Could you check a few things on this model? Use its own coordinates, in mm. Face numbers are marked on the shaded views. A direction names the side the tool comes from. Give positions to 0.01 mm unless a question says otherwise; leave off trailing zeros. Write each loop counter-clockwise with the first axis right and the second up, starting at its lowest first coordinate (ties: lowest second). Pieces come first, ordered by that corner, then holes. Notation, with made-up numbers: (82, 20.5) - (96, 20.5) arc R26 cw to (96, 47.5) - close; hole circle Ø5 at (33, -4.5). An arc over 180 degrees is marked (long way). Answer as CSV lines item,"result". Start each with the question number.
Q1. Will these pins go through, and if not, where does the flat tip stop? pin 1 Ø1.5 at (x, z) = (2.5, 4) entering from +Y; pin 2 Ø2 at (x, z) = (9.5, 3.5) entering from +Y; pin 3 Ø2 at (x, z) = (11.5, 14) entering from -Y.
Q2. Imagine slicing it at C-C on z = 22.5. List the corners of the cut face in (x, y) for me, and give its area (3 significant figures).
Q3. On a 3-axis mill with a long thin cutter (end or side, diameter ignored), from which of +Z, -Z, +X, -X, +Y, -Y can I reach the whole of each face in a straight line? I mean the marked faces 4, 5 and 6. Say none if no direction works.
Q4. We'd pull the mould along Y, two halves only. Please class the marked faces 1, 2 and 3: pulls with the +Y half, pulls with the -Y half, needs draft (parallel to the pull), parting line crosses it, or undercut.
Q5. Imagine slicing it at A-A on z = 10.5. List the corners of the cut face in (x, y) for me.
Q6. Imagine slicing it at D-D on x = 8.5. List the corners of the cut face in (y, z) for me, and give its area (3 significant figures).
Q7. If I drill on line 1 along Y through (x, z) = (0, 4); line 2 along X through (y, z) = (0, 5); line 3 along Y through (x, z) = (-5, 19.25), over which ranges is the centre line in solid material (lowest first)?
```python
from build123d import *

# Parameters (mm, degrees)
F0_R     = 15
F1_DEPTH = 9
F2_R     = 0.5
F3_DEPTH = 10
F6_DEPTH = 5


# Not quite as in the source:
# - a fillet or chamfer that OpenCascade refuses, or shapes differently, is made with other operations: its cross-section is extruded or revolved along the edge and cut away or added


with BuildPart() as f1:
    # F0 (on Top) → F1 (new body)
    with BuildSketch(Plane.XY):
        Circle(F0_R)
        with BuildLine():
            Line((-2.2, -2.3237900077), (-2.2, 2.3237900077))
            ThreePointArc((-2.2, 2.3237900077), (3.2, 0), (-2.2, -2.3237900077))
        make_face(mode=Mode.SUBTRACT)
    extrude(amount=F1_DEPTH)

    # F2 (on face) → F3 (join)
    with BuildSketch(Plane.XY.offset(9)):
        with BuildLine():
            Line((-7, 6), (-15, 0))
            Line((-15, 0), (-7, -6))
            Line((-7, -6), (13.7477270849, -6))
            ThreePointArc((13.7477270849, -6), (14.683594694, -3.0646446553), (15, 0))
            ThreePointArc((15, 0), (14.683594694, 3.0646446553), (13.7477270849, 6))
            Line((13.7477270849, 6), (-7, 6))
        make_face()
        Circle(F2_R, mode=Mode.SUBTRACT)
    extrude(amount=F3_DEPTH)

    # F4: chamfer of 10 x 2.6794919243 on 1 edges, made by hand


with BuildPart() as f4_tool2:
    # F4_s3 → F4_t4 (revolve)
    with BuildSketch(Plane.XZ):
        Polygon((3.1794919243, 9), (0.5, 19), (0.5, 9), align=None)
    revolve(axis=Axis((0, 0, 9), (0, 0, 1)))

    split(bisect_by=Plane.YZ.offset(-2.2), keep=Keep.TOP)


with BuildPart() as f1_1:
    add(f1.part)

    # F4_t1: cut F4_tool2
    add(f4_tool2.part, mode=Mode.SUBTRACT)

    # F5 (on face) → F6 (join)
    with BuildSketch(Plane.XY.offset(19)):
        with BuildLine():
            Line((-7, 6), (-15, 0))
            Line((-15, 0), (-7, -6))
            Line((-7, -6), (13.7477270849, -6))
            ThreePointArc((13.7477270849, -6), (15, 0), (13.7477270849, 6))
            Line((13.7477270849, 6), (-7, 6))
        make_face()
    extrude(amount=F6_DEPTH)


solid = f1_1.part
```
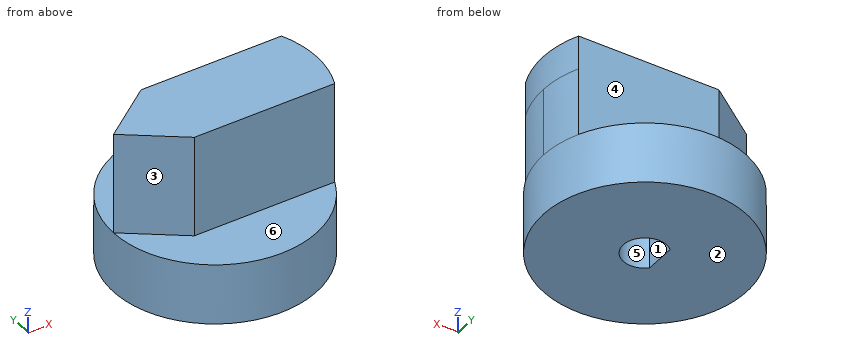
Conclusion:
1,pin 1,"y = 14.9"
1,pin 2,"y = 12.36"
1,pin 3,"y = -6"
2,outline,"(-15, 0) - (-7, -6) - (13.75, -6) arc R15 ccw to (13.75, 6) - (-7, 6) - close"
2,area,"307 mm^2"
3,face 4,"+Z, +X, -X, +Y"
3,face 5,"-Z"
3,face 6,"+Z, -X, -Y"
4,face 1,"undercut"
4,face 2,"needs draft"
4,face 3,"pulls with the -Y half"
5,outline,"(-15, 0) - (-7, -6) - (13.75, -6) arc R15 ccw to (13.75, 6) - (-7, 6) - close; hole (-2.2, -1.7) arc R2.78 ccw (long way) to (-2.2, 1.7) - close"
6,outline,"(-12.36, 0) - (12.36, 0) - (12.36, 9) - (6, 9) - (6, 24) - (-6, 24) - (-6, 9) - (-12.36, 9) - close"
6,area,"402 mm^2"
7,line 1,"-15 to -3.2, 3.2 to 15"
7,line 2,"-15 to -2.2, 3.2 to 15"
7,line 3,"-6 to 6"
